Geometry: final body of the model. Coordinates: model frame, mm. A direction names the side the tool comes from. Coordinates: 2 decimals unless noted, no trailing zeros. Order: outer loops, then holes, each group sorted by start corner. A loop starts at its lowest first (then second) coordinate and runs counter-clockwise, first axis right, second up. Notation, with made-up numbers: (61.5, 35.25) - (68.5, 35.25) arc R14 ccw to (68.5, 61.25) - close; hole circle Ø8 at (64.25, 18). An arc over 180 degrees is marked (long way). Use a Markdown table: item, result. Add a question column.
```python
from build123d import *

# Parameters (mm, degrees)
AXLE_BASE_SKETCH_R        = 25.5
AXLE_DEPTH                = 68.5
GUARD_BASE_R              = 37.5
GUARD_DEPTH               = 5
INNER_AXLE_HOLE_BASE_R    = 8.5
INNER_AXLE_HOLE_DEPTH     = 74.5
BEND_START                = -56.5
BEND_ROOM_BASE_W          = 1.5
BEND_ROOM_BASE_H          = 75
BEND_ROOM_1_DEPTH         = 56.500001
BEND_ROOM_2_COUNT         = 2
BEND_ROOM_2_ANGLE         = 90
EASY_REMOVAL_CHAMFER_SIZE = 4


with BuildPart() as part:
    # Axle base sketch → Axle (new body)
    with BuildSketch(Plane.XY):
        Circle(AXLE_BASE_SKETCH_R)
    extrude(amount=AXLE_DEPTH)

    # Guard base → Guard (add)
    with BuildSketch(Plane(origin=(0, 0, 0), x_dir=(-1, 0, 0), z_dir=(0, 0, -1))):
        Circle(GUARD_BASE_R)
    extrude(amount=GUARD_DEPTH)

    # Inner axle hole base → Inner axle hole (cut, through all)
    with BuildSketch(Plane.XY.offset(68.5)):
        Circle(INNER_AXLE_HOLE_BASE_R)
    extrude(amount=-INNER_AXLE_HOLE_DEPTH, mode=Mode.SUBTRACT)

    # Mate ring base → Mate rings (revolve)
    with BuildSketch(Plane(origin=(0, 0, 0), x_dir=(1, 0, 0), z_dir=(0, 1, 0))):
        Polygon((25.5, -68.5), (26.25, -67.75), (26.25, -67), (25.5, -66.25), align=None)
        Polygon((25.5, -62.75), (26.25, -62), (26.25, -61.25), (25.5, -60.5), align=None)
    revolve(axis=Axis((0, 0, 0), (0, 0, -1)))

    # Inner mass remove base → Inner mass remove (revolve, cut)
    with BuildSketch(Plane(origin=(0, 0, 0), x_dir=(0, 0, -1), z_dir=(1, 0, 0))):
        Polygon((-68.5, 0), (-51.5, -17), (-12, -17), (5, 0), align=None)
    revolve(axis=Axis((0, 0, 0), (0, 0, -1)), mode=Mode.SUBTRACT)

    # Bend room base → Bend room 1 (cut)
    with BuildSketch(Plane.XY.offset(68.5).offset(BEND_START)):
        Rectangle(BEND_ROOM_BASE_W, BEND_ROOM_BASE_H)
    bend_room_1 = extrude(amount=BEND_ROOM_1_DEPTH, mode=Mode.SUBTRACT)

    # Bend room 2: Bend room 1 ×2 about axis
    bend_room_2_axis = Axis((0, 0, 0), (0, 0, -1))
    for i in range(1, BEND_ROOM_2_COUNT):
        add(bend_room_1.rotate(bend_room_2_axis, i * BEND_ROOM_2_ANGLE / (BEND_ROOM_2_COUNT - 1)), mode=Mode.SUBTRACT)

    # Easy removal chamfer
    easy_removal_chamfer_edges = [part.edges().sort_by_distance(p)[0] for p in [
        (37.5, 0, 0),
    ]]
    chamfer(easy_removal_chamfer_edges, length=EASY_REMOVAL_CHAMFER_SIZE)


solid = part.part
```
1) Set-up query: faces 1 (the face through (-18.76, 18.36, 61.62)), 2 (the face through (-6.07, -5.95, 64.31)), 3 (the face through (18.31, -17.92, 60.62)), 4 (the face through (-2.68, -8.5, 3.91)), 5 (the face through (-18.31, 17.92, 66.37)). Return all of +Z, -Z, +X, -X, +Y, -Y with unobstructed straight access to the full face (end or side cutting, diameter ignored); none if empty.
2) Ray query, line 1 along X through (y, z) = (0, 0.25); line 2 along Y through (x, z) = (0, -2); line 3 along X through (y, z) = (-20, 38). Return the intervals inside material, ascending.
3) Pin query (flat end, axial travel): pin 1 (6 mm diameter, centred on y = 7.5, z = 36.5, fed in from +X); pin 2 (0.8 mm diameter, centred on x = -21.5, y = 0, fed in from +Z); pin 3 (5.5 mm diameter, centred on y = -17, z = 49, fed in from +X); pin 4 (10 mm diameter, centred on x = 0, y = 0, fed in from -Z). Return the tip coordinate at first contact, or that it passes through.
4) Section A-A (z = 15.5). Return loops of the section in (x, y).
5) Draft query along X for faces 6 (the face through (6.07, 5.95, 64.31)), 7 (the face through (18.314, -17.93, 62.62)), 8 (the face through (13, -13, 68.5)). Return one class per face: pulls with the +X half, pulls with the -X half, needs draft (parallel to the pull), parting line crosses it, or undercut.
Values follow:
| question | item | result |
|---|---|---|
| 1 | face 1 | +Z, -X, +Y |
| 1 | face 2 | +Z, -Z |
| 1 | face 3 | +X, -Y |
| 1 | face 4 | none |
| 1 | face 5 | -X, +Y |
| 2 | line 1 | x = -25.5 to -8.5, 8.5 to 25.5 |
| 2 | line 2 | y = -35.5 to -8.5, 8.5 to 35.5 |
| 2 | line 3 | x = -15.82 to -0.75, 0.75 to 15.82 |
| 3 | pin 1 | stops at x = 25.1 |
| 3 | pin 2 | stops at z = 12 |
| 3 | pin 3 | stops at x = 21.15 |
| 3 | pin 4 | passes through |
| 4 | outline | (-25.49, -0.75) arc R25.5 ccw to (-0.75, -25.49) - (-0.75, -16.98) arc R17 cw to (-16.98, -0.75) - close; (-25.49, 0.75) - (-16.98, 0.75) arc R17 cw to (-0.75, 16.98) - (-0.75, 25.49) arc R25.5 ccw to start; (0.75, -25.49) arc R25.5 ccw to (25.49, -0.75) - (16.98, -0.75) arc R17 cw to (0.75, -16.98) - close; (0.75, 16.98) arc R17 cw to (16.98, 0.75) - (25.49, 0.75) arc R25.5 ccw to (0.75, 25.49) - close |
| 5 | face 6 | undercut |
| 5 | face 7 | pulls with the +X half |
| 5 | face 8 | needs draft |
